Can you work these out from the model? Positions are in its coordinate system, mm. A direction names the side the tool comes from. Coordinates: 2 decimals unless noted, no trailing zeros. Answer as a JSON object with one key per item and string values. Group by question number.
from build123d import *

# Parameters (mm, degrees)
SKETCH1_W           = 609.6
SKETCH1_H           = 152.4
SKETCH1_R           = 2.246
SKETCH1_R_2         = 4.5085
BOSS_EXTRUDE1_DEPTH = 12.7


with BuildPart() as part:
    # Sketch1 → Boss-Extrude1 (new body)
    with BuildSketch(Plane.XY):
        Rectangle(SKETCH1_W, SKETCH1_H)
        with Locations((53, 68.1999984)):
            Circle(SKETCH1_R, mode=Mode.SUBTRACT)
        with Locations((82.698486542, 55.898482492)):
            Circle(SKETCH1_R, mode=Mode.SUBTRACT)
        with Locations((95.00000245, 26.19999595)):
            Circle(SKETCH1_R, mode=Mode.SUBTRACT)
        with Locations((82.698486542, -3.498490592)):
            Circle(SKETCH1_R, mode=Mode.SUBTRACT)
        with Locations((23.301513458, -3.498490592)):
            Circle(SKETCH1_R, mode=Mode.SUBTRACT)
        with Locations((10.99999755, 26.19999595)):
            Circle(SKETCH1_R, mode=Mode.SUBTRACT)
        with Locations((23.301513458, 55.898482492)):
            Circle(SKETCH1_R, mode=Mode.SUBTRACT)
        with Locations((238.76, 63.5)):
            Circle(SKETCH1_R_2, mode=Mode.SUBTRACT)
        with Locations((200.66, 63.5)):
            Circle(SKETCH1_R_2, mode=Mode.SUBTRACT)
        with Locations(Location((238.76, -63.5, 0), (0, 0, 180))):
            Circle(SKETCH1_R_2, mode=Mode.SUBTRACT)
        with Locations(Location((200.66, -63.5, 0), (0, 0, 180))):
            Circle(SKETCH1_R_2, mode=Mode.SUBTRACT)
        with Locations(Location((-82.698486542, -3.498490592, 0), (0, 0, 180))):
            Circle(SKETCH1_R, mode=Mode.SUBTRACT)
        with Locations(Location((-95.00000245, 26.19999595, 0), (0, 0, 180))):
            Circle(SKETCH1_R, mode=Mode.SUBTRACT)
        with Locations(Location((-82.698486542, 55.898482492, 0), (0, 0, 180))):
            Circle(SKETCH1_R, mode=Mode.SUBTRACT)
        with Locations(Location((-53, 68.1999984, 0), (0, 0, 180))):
            Circle(SKETCH1_R, mode=Mode.SUBTRACT)
        with Locations(Location((-23.301513458, 55.898482492, 0), (0, 0, 180))):
            Circle(SKETCH1_R, mode=Mode.SUBTRACT)
        with Locations(Location((-10.99999755, 26.19999595, 0), (0, 0, 180))):
            Circle(SKETCH1_R, mode=Mode.SUBTRACT)
        with Locations(Location((-23.301513458, -3.498490592, 0), (0, 0, 180))):
            Circle(SKETCH1_R, mode=Mode.SUBTRACT)
        with Locations(Location((-238.76, 63.5, 0), (0, 0, 180))):
            Circle(SKETCH1_R_2, mode=Mode.SUBTRACT)
        with Locations(Location((-200.66, 63.5, 0), (0, 0, 180))):
            Circle(SKETCH1_R_2, mode=Mode.SUBTRACT)
        with Locations((-200.66, -63.5)):
            Circle(SKETCH1_R_2, mode=Mode.SUBTRACT)
        with Locations((-238.76, -63.5)):
            Circle(SKETCH1_R_2, mode=Mode.SUBTRACT)
        with BuildLine():
            Line((34.25, -6.275954242), (34.25, -25.4))
            Line((34.25, -25.4), (71.75, -25.4))
            Line((71.75, -25.4), (71.75, -6.275954242))
            ThreePointArc((71.75, -6.275954242), (53, 63.6999984), (34.25, -6.275954242))
        make_face(mode=Mode.SUBTRACT)
        with BuildLine():
            Line((-34.25, -6.275954242), (-34.25, -25.4))
            Line((-34.25, -25.4), (-71.75, -25.4))
            Line((-71.75, -25.4), (-71.75, -6.275954242))
            ThreePointArc((-71.75, -6.275954242), (-53, 63.6999984), (-34.25, -6.275954242))
        make_face(mode=Mode.SUBTRACT)
    extrude(amount=BOSS_EXTRUDE1_DEPTH)


solid = part.part
Q1. If we section it at A-A on z = 3.25: Give the number of separate pieces and of enclosed holes in the cut face, and give its area (3 significant figures).
Q2. Will this pin go through, and if not, where does the flat tip stop? pin 1 (8 mm diameter, centred on x = -238.76, y = 63.5, fed in from +Z).
Q3. On a 3-axis mill with a long thin cutter (end or side, diameter ignored), from which of +Z, -Z, +X, -X, +Y, -Y can I reach the whole of each face in a straight line? I mean faces 5 (the flat face through (-4, 1, 0)), 6 (the flat face through (-71.75, -16, 6)). Say none if no direction works.
Q4. Please list where these lines run through material, in increasing order: L1, parallel to Y at x = 200.66, z = 7; L2, parallel to X at y = 23.5, z = 3; L3, parallel to Y at x = 94.5, z = 9.
Q5. We'd pull the mould along X, two halves only. Please class faces 1 (the flat face through (-304.8, -1, 6)), 2 (the flat face through (-4, -76.2, 6)), 3 (the cylindrical face through (-54.374, 63.675, 6.261)), 4 (the flat face through (304.8, -1, 6)): pulls with the +X half, pulls with the -X half, needs draft (parallel to the pull), parting line crosses it, or undercut.
Reply:
{
 "1": {"separate pieces": "1", "enclosed holes": "24", "area": "82,200 mm^2"},
 "2": {"pin 1": "through"},
 "3": {"face 5": "-Z, +X, -X, +Y, -Y", "face 6": "+Z, -Z"},
 "4": {"L1": "-76.2 to -68.01, -58.99 to 58.99, 68.01 to 76.2", "L2": "-304.8 to -90.4, -15.6 to 15.6, 90.4 to 304.8", "L3": "-76.2 to 24.01, 28.39 to 76.2"},
 "5": {"face 1": "pulls with the -X half", "face 2": "needs draft", "face 3": "undercut", "face 4": "pulls with the +X half"}
}
